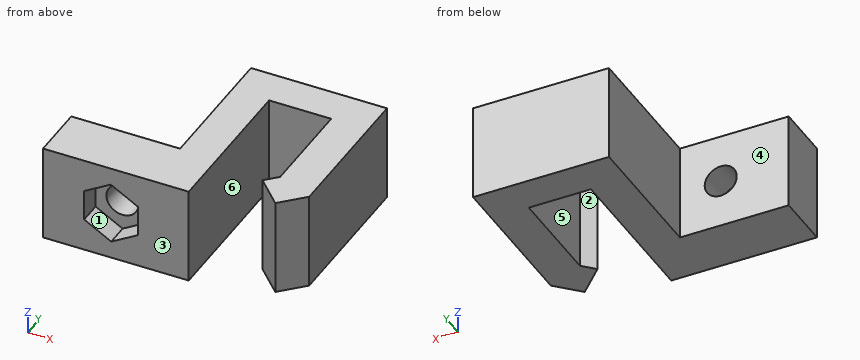
from build123d import *

# Parameters (mm, degrees)
F1_DEPTH = 10
F2_R     = 1.65
F4_DEPTH = 20.001
F5_DEPTH = 2.3


with BuildPart() as f1:
    # F0 (on Top) → F1 (new body)
    with BuildSketch(Plane.XY):
        Polygon((0, 5.7), (0, 0), (15, 0), (15, 16.2), (21.4, 16.2), (21.4, 5.8870057685), (20.2, 4.6870057685), (22.8870057685, 2), (25.2, 4.3129942315), (25.2, 20), (11.2, 20), (11.2, 5.7), align=None)
    extrude(amount=F1_DEPTH)

    # F2 (on face) → F4 (cut, through all)
    with BuildSketch(Plane.XZ):
        with Locations((7, 5)):
            Circle(F2_R)
    extrude(amount=-F4_DEPTH, mode=Mode.SUBTRACT)

    # F2 (on face) → F5 (cut)
    with BuildSketch(Plane.XZ):
        Polygon((6.9812222395, 8.1999449051), (4.2193775412, 6.5837104349), (4.2381553017, 3.3837655298), (7.0187777605, 1.8000550949), (9.7806224588, 3.4162895651), (9.7618446983, 6.6162344702), align=None)
        with Locations((7, 5)):
            Circle(F2_R, mode=Mode.SUBTRACT)
    extrude(amount=-F5_DEPTH, mode=Mode.SUBTRACT)


solid = f1.part
Build history of the part. All positions in model axes, mm. Face numbers are marked on the shaded views. A direction names the side the tool comes from. Give positions to 0.01 mm unless a question says otherwise; leave off trailing zeros. Order: outer loops, then holes, each group sorted by start corner. A loop starts at its lowest first (then second) coordinate and runs counter-clockwise, first axis right, second up. Notation, with made-up numbers: M 3.25,72.5 L 17.25,72.5 A19 cw 17.25,85.5 Z; hole C 25.5,-14.75 d4. An arc over 180 degrees is marked long. Use one line per item in the form item = value.
1) Probe probe 1 along X at (y, z) = (11, 9.5); probe 2 along Z at (x, y) = (7, 3.9); probe 3 along Y at (x, z) = (19, 6.75). List the from-to ranges inside material, lowest first.
Calculated:
probe_1 = 11.2 to 15, 21.4 to 25.2
probe_2 = 0 to 3.35, 6.65 to 10
probe_3 = 16.2 to 20
2) Saw through at B-B (z = 5.75). Give the cut face in (x, y).
Calculated:
outline = M 0,0 L 4.22,0 L 4.22,2.3 L 5.53,2.3 L 5.53,5.7 L 0,5.7 Z; M 8.47,2.3 L 9.77,2.3 L 9.77,0 L 15,0 L 15,16.2 L 21.4,16.2 L 21.4,5.89 L 20.2,4.69 L 22.89,2 L 25.2,4.31 L 25.2,20 L 11.2,20 L 11.2,5.7 L 8.47,5.7 Z
3) Drop flat-ended pins along their axis: pin 1 (3 mm diameter, centred on x = 19.5, z = 7.5, fed in from -Y); pin 2 (1 mm diameter, centred on y = 16.5, z = 1.5, fed in from -X); pin 3 (3 mm diameter, centred on x = 3.5, z = 3.5, fed in from +Y). Give the stop position or say it passes through.
Calculated:
pin_1 = 3.89
pin_2 = 11.2
pin_3 = 5.7
4) Tool access for the marked faces 4, 5 and 6: list every direction of +Z, -Z, +X, -X, +Y, -Y with a clear straight run to the whole face (end or side of a thin tool).
Calculated:
face_4 = +Z, -Z, -X, +Y
face_5 = +Z, -Z
face_6 = +Z, -Z, -Y
5) Saw through at C-C (x = 5.75). Give the cut face in (y, z).
Calculated:
outline = M 0,0 L 5.7,0 L 5.7,3.92 L 2.3,3.92 L 2.3,2.52 L 0,2.52 Z; M 0,7.48 L 2.3,7.48 L 2.3,6.08 L 5.7,6.08 L 5.7,10 L 0,10 Z
6) Two-plate mould, pull along Y, no slides. Class the marked faces 1, 2 and 3: released by +Y, released by -Y, zero draft, split by the parting line, or undercut.
Calculated:
face_1 = zero draft
face_2 = undercut
face_3 = released by -Y
7) Saw through at D-D (y = 18.75). Give the cut face in (x, z).
Calculated:
outline = M 11.2,0 L 25.2,0 L 25.2,10 L 11.2,10 Z
8) Saw through at A-A (y = 11.25). Give the cut face in (x, z), plus the area to 3 significant figures.
Calculated:
outline = M 11.2,0 L 15,0 L 15,10 L 11.2,10 Z; M 21.4,0 L 25.2,0 L 25.2,10 L 21.4,10 Z
area = 76.0 mm2
